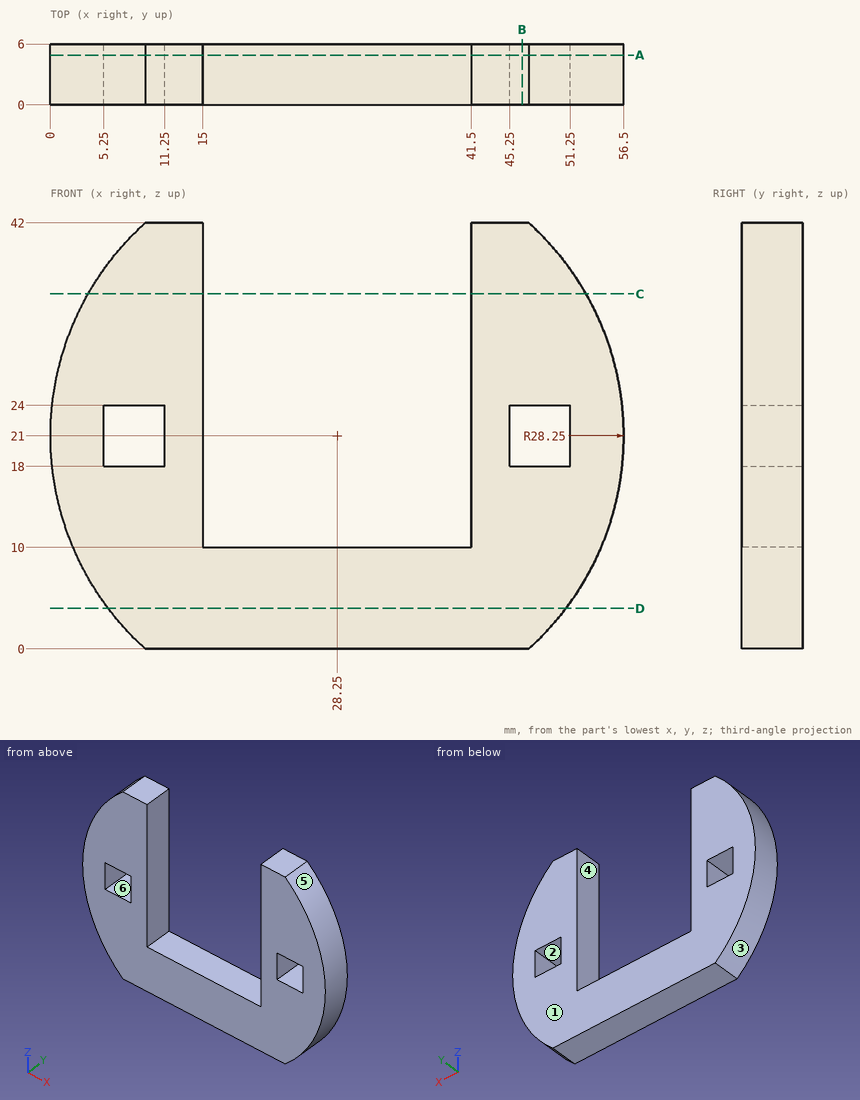
Design review of the part shown in the three views and the two pictorial views. Dimensions are in mm from the part's minimum x, y and z. A direction names the side the tool comes from. Coordinates: 2 decimals unless noted, no trailing zeros. Loops run counter-clockwise (first coordinate to the right, second up) from the corner with the lowest first, then second, coordinate; pieces in that order, holes last. Notation, with made-up numbers: M 53.25,5 L 67.25,5 A21 cw 67.25,41 Z; hole C 36,-28.75 d3. An arc over 180 degrees is marked long. Put each result on its own line as item: value. Start each with the question number.
Q1. Add section B-B (x = 46.5). Write out the cut boundary in (y, z), and give its area (3 significant figures).
Q2. For the marked faces 4, 5 and 6, list the 3-axis set-ups (+Z, -Z, +X, -X, +Y, -Y) from which the entire face can be reached by the end or side of a thin tool; tool diameter is ignored.
Q3. Wall thickness on line 1 (X direction, y = 1.5, z = 19); line 2 (Z direction, x = 10, y = 2.7); line 3 (Z direction, x = 30, y = 0.9): over which ranges is each line inside the solid? List them lowest first.
Q4. Add section D-D (z = 4). Write out the cut boundary in (x, y), and give its area (3 significant figures).
Q5. Add section A-A (y = 4.9). Write out the cut boundary in (x, z), and give its area (3 significant figures).
Q6. The part is to be moulded in two halves that separate along Z. For the marked faces 1, 2 and 3, say which applies: +Z half, -Z half, draft (parallel to the pull), parting line (faces both ways), or undercut.
Q7. Add section C-C (z = 35). Write out the cut boundary in (x, y), and give its area (3 significant figures).
Q8. Clearance check with flat-ended pins moving along their axes: pin 1 (1 mm diameter, centred on x = 31, y = 1, fed in from +Z); pin 2 (3 mm diameter, centred on y = 5, z = 30.5, fed in from +X); pin 3 (1.8 mm diameter, centred on y = 4.5, z = 19.5, fed in from -X). State where each tip first meets the part, or that it passes through.
Answers:
1. outline: M 0,0 L 6,0 L 6,18 L 0,18 Z; M 0,24 L 6,24 L 6,42 L 0,42 Z
1. area: 216 mm^2
2. face 4: +Z, +Y, -Y
2. face 5: +X, +Y, -Y
2. face 6: +Y, -Y
3. line 1: x = 0.07 to 5.25, 11.25 to 15, 41.5 to 45.25, 51.25 to 56.43
3. line 2: z = 0 to 18, 24 to 42
3. line 3: z = 0 to 10
4. outline: M 5.69,0 L 50.81,0 L 50.81,6 L 5.69,6 Z
4. area: 271 mm^2
5. outline: M 9.35,0 L 47.15,0 A28.25 ccw 47.15,42 L 41.5,42 L 41.5,10 L 15,10 L 15,42 L 9.35,42 A28.25 ccw Z; hole M 5.25,18 L 11.25,18 L 11.25,24 L 5.25,24 Z; hole M 45.25,18 L 51.25,18 L 51.25,24 L 45.25,24 Z
5. area: 1,210 mm^2
6. face 1: draft
6. face 2: undercut
6. face 3: parting line
7. outline: M 3.71,0 L 15,0 L 15,6 L 3.71,6 Z; M 41.5,0 L 52.79,0 L 52.79,6 L 41.5,6 Z
7. area: 135 mm^2
8. pin 1: stops at z = 10
8. pin 2: stops at x = 55.34
8. pin 3: stops at x = 0.01
